from build123d import *

# Parameters (mm, degrees)
CYLINDER038_R            = 1.8
CYLINDER038_DEPTH        = 100
ARRAY001_X_COUNT         = 2
ARRAY001_X_PITCH         = 25
ARRAY001_Y_COUNT         = 2
ARRAY001_Y_PITCH         = 11
ARRAY001_PLACEMENT_ANGLE = 90
ARRAY002_Z_COUNT         = 2
ARRAY002_Z_PITCH         = 80
SKETCH001_W              = 43.249981
SKETCH001_H              = 25.364647
SKETCH001_W_2            = 44.875929
SKETCH001_H_2            = 23.738708
EXTRUDE001_DEPTH         = 50
CYLINDER011002_R         = 1.8
CYLINDER011002_DEPTH     = 100
ARRAY004_X_COUNT         = 9
ARRAY004_X_PITCH         = 10
ARRAY004_Z_COUNT         = 9
ARRAY004_Z_PITCH         = 10
BOX001_W                 = 97
BOX001_H                 = 3
BOX001_DEPTH             = 100
FILLET001_R              = 2


with BuildPart() as bolt_hole_array_pair:
    # Cylinder038 → Cylinder038 (new body)
    with BuildSketch(Plane.XY.offset(-50)):
        Circle(CYLINDER038_R)
    extrude(amount=CYLINDER038_DEPTH)

    # Array001 X: bolt hole array pair ×2


with BuildPart() as bolt_hole_array_pair_1:
    add(bolt_hole_array_pair.part)
    with Locations(*[(i * ARRAY001_X_PITCH, 0, 0) for i in range(1, ARRAY001_X_COUNT)]):
        add(bolt_hole_array_pair.part)

    # Array001 Y: bolt hole array pair ×2


with BuildPart() as bolt_hole_array_pair_2:
    add(bolt_hole_array_pair_1.part)
    with Locations(*[(0, i * ARRAY001_Y_PITCH, 0) for i in range(1, ARRAY001_Y_COUNT)]):
        add(bolt_hole_array_pair_1.part)


with BuildPart() as bolt_hole_array_pair_3:
    # Array001 placement: moved
    add(bolt_hole_array_pair_2.part.moved(Location((-12.5, 0, 4.5))).rotate(Axis((-12.5, 0, 4.5), (1, 0, 0)), ARRAY001_PLACEMENT_ANGLE))

    # Array002 Z: bolt hole array pair ×2


with BuildPart() as bolt_hole_array_pair_4:
    add(bolt_hole_array_pair_3.part)
    with Locations(*[(0, 0, i * ARRAY002_Z_PITCH) for i in range(1, ARRAY002_Z_COUNT)]):
        add(bolt_hole_array_pair_3.part)


with BuildPart() as pulley_side_extrude:
    # Sketch001 (on Array) → Extrude001 (new body, symmetric)
    with BuildSketch(Plane(origin=(-14.5, 0, 10), x_dir=(1, 0, 0), z_dir=(0, -1, 0))):
        with Locations((13.668077, 77.054226)):
            Rectangle(SKETCH001_W, SKETCH001_H)
        with Locations((13.180285, 1.773257)):
            Rectangle(SKETCH001_W_2, SKETCH001_H_2)
    extrude(amount=EXTRUDE001_DEPTH, both=True)


with BuildPart() as pulley_side_hole_fusion:
    # Cylinder011002 → Cylinder011002 (new body)
    with BuildSketch(Plane.XZ.offset(-50)):
        Circle(CYLINDER011002_R)
    extrude(amount=CYLINDER011002_DEPTH)

    # Array004 X: pulley side hole fusion ×9


with BuildPart() as pulley_side_hole_fusion_1:
    add(pulley_side_hole_fusion.part)
    with Locations(*[(i * ARRAY004_X_PITCH, 0, 0) for i in range(1, ARRAY004_X_COUNT)]):
        add(pulley_side_hole_fusion.part)

    # Array004 Z: pulley side hole fusion ×9


with BuildPart() as pulley_side_hole_fusion_2:
    add(pulley_side_hole_fusion_1.part)
    with Locations(*[(0, 0, i * ARRAY004_Z_PITCH) for i in range(1, ARRAY004_Z_COUNT)]):
        add(pulley_side_hole_fusion_1.part)


with BuildPart() as pulley_side_hole_fusion_3:
    # Array004 placement: moved
    add(pulley_side_hole_fusion_2.part.moved(Location((-14.5, 0, 10))))

    # Cut023015009003: cut pulley side extrude
    add(pulley_side_extrude.part, mode=Mode.SUBTRACT)

    # Fusion001: union bolt hole array pair
    add(bolt_hole_array_pair_4.part)


with BuildPart() as pulley_side_plate_cut:
    # Box001 → Box001 (new body)
    with BuildSketch(Plane(origin=(-23, 33, 0), x_dir=(1, 0, 0), z_dir=(0, 0, 1))):
        with Locations((48.5, 1.5)):
            Rectangle(BOX001_W, BOX001_H)
    extrude(amount=BOX001_DEPTH)

    # Fillet001
    fillet001_edges = [pulley_side_plate_cut.edges().sort_by_distance(p)[0] for p in [
        (-23, 34.5, 100),
        (-23, 34.5, 0),
        (74, 34.5, 100),
        (74, 34.5, 0),
    ]]
    fillet(fillet001_edges, radius=FILLET001_R)

    # Cut023015009004: cut pulley side hole fusion
    add(pulley_side_hole_fusion_3.part, mode=Mode.SUBTRACT)


solid = pulley_side_plate_cut.part
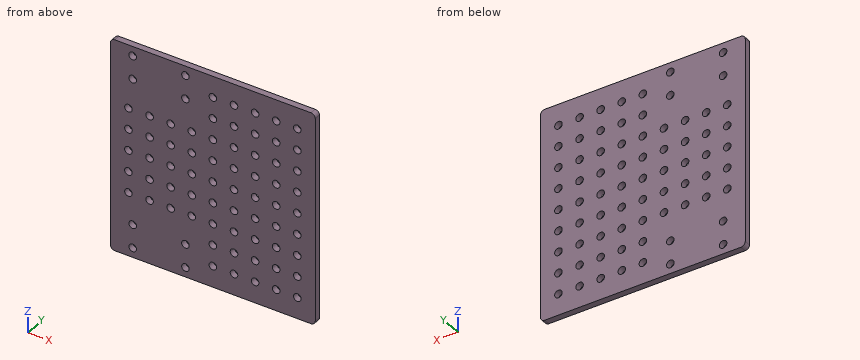
Could you check a few things on this model? Use its own coordinates, in mm. Coordinates: 2 decimals unless noted, no trailing zeros. Order: outer loops, then holes, each group sorted by start corner. A loop starts at its lowest first (then second) coordinate and runs counter-clockwise, first axis right, second up. Notation, with made-up numbers: (8, -32) - (59, -32) arc R20 cw to (59, -17) - close; hole circle Ø3 at (-25.5, 2). An arc over 180 degrees is marked (long way). Answer in a Markdown table with one row per item. Add a question column.
(1) If we section it at A-A, the plane z = 80: Please give me the cut outline in (x, y).
(2) I need wall thicknesses on L1, parallel to X at y = 34.3, z = 90; L2, parallel to X at y = 33.7, z = 15.5; L3, parallel to X at y = 33.45, z = 78.5. Which ranges of each line are inside material? Lowest first, please.
(3) If we section it at B-B, the plane y = 35.15: State how many separate pieces and enclosed holes the cut face has, then the cut area to 3 significant figures.
Results are:
| question | item | result |
|---|---|---|
| 1 | outline | (-23, 33) - (23.7, 33) - (23.7, 36) - (-23, 36) - close; (27.3, 33) - (33.7, 33) - (33.7, 36) - (27.3, 36) - close; (37.3, 33) - (43.7, 33) - (43.7, 36) - (37.3, 36) - close; (47.3, 33) - (53.7, 33) - (53.7, 36) - (47.3, 36) - close; (57.3, 33) - (63.7, 33) - (63.7, 36) - (57.3, 36) - close; (67.3, 33) - (74, 33) - (74, 36) - (67.3, 36) - close |
| 2 | L1 | x = -23 to 23.7, 27.3 to 33.7, 37.3 to 43.7, 47.3 to 53.7, 57.3 to 63.7, 67.3 to 74 |
| 2 | L2 | x = -23 to -14.3, -10.7 to 10.7, 14.3 to 74 |
| 2 | L3 | x = -23 to 24.51, 26.49 to 34.51, 36.49 to 44.51, 46.49 to 54.51, 56.49 to 64.51, 66.49 to 74 |
| 3 | separate pieces | 1 |
| 3 | enclosed holes | 73 |
| 3 | area | 8,950 mm2 |
